```python
from build123d import *

# Parameters (mm, degrees)
F0_W     = 203.2
F0_H     = 127
F1_DEPTH = 127
F2_R     = 5.08
F3_W     = 152.4
F3_H     = 114.3
F4_DEPTH = 101.6
F3_W_2   = 31.75
F5_DEPTH = 6.35


with BuildPart() as f1:
    # F0 (on Top) → F1 (new body)
    with BuildSketch(Plane.XY):
        with Locations((38.395604, 24.034617)):
            Rectangle(F0_W, F0_H)
    extrude(amount=F1_DEPTH)

    # F2
    f2_edges = [f1.edges().sort_by_distance(p)[0] for p in [
        (38.395604, -39.465383, 127),
        (-63.204396, 24.034617, 127),
        (139.995604, 24.034617, 127),
        (139.995604, -39.465383, 63.5),
        (-63.204396, -39.465383, 63.5),
    ]]
    fillet(f2_edges, radius=F2_R)

    # F3 (on face) → F4 (cut)
    with BuildSketch(Plane.XZ.offset(39.465383)):
        with Locations((56.842002, 63.221574)):
            Rectangle(F3_W, F3_H)
    extrude(amount=-F4_DEPTH, mode=Mode.SUBTRACT)

    # F3 (on face) → F5 (cut)
    with BuildSketch(Plane.XZ.offset(39.465383)):
        with Locations((56.842002, 63.221574)):
            Rectangle(F3_W, F3_H)
        with Locations((-39.926485, 63.221574)):
            Rectangle(F3_W_2, F3_H)
    extrude(amount=-F5_DEPTH, mode=Mode.SUBTRACT)


solid = f1.part
```
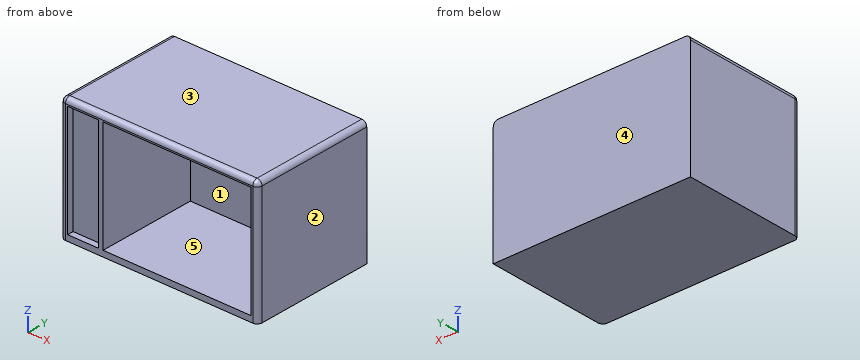
Check sheet for the modelled part. Datum: model origin and axes. Units: mm. Face numbers are marked on the shaded views. A direction names the side the tool comes from. Give positions to 0.01 mm unless a question says otherwise; leave off trailing zeros. Order: outer loops, then holes, each group sorted by start corner. A loop starts at its lowest first (then second) coordinate and runs counter-clockwise, first axis right, second up. Notation, with made-up numbers: (-2, 49.5) -> (47, 49.5) arc R31 cw to (47, 85.5) -> close; hole circle Ø8 at (79, 69.25). An arc over 180 degrees is marked (long way). Use CSV: the item, a comma, the result in double quotes. Start each with the question number.
1) Mould release check, pull along Z, two halves, no side actions. Record for the marked faces 1, 2 and 3: released by +Z, released by -Z, zero draft, split by the parting line, or undercut.
2) Sectioned sample at B-B, the plane x = -38. Record the boundary of the cut face in (y, z).
3) Go/stop test with flat-tipped pins: P1, Ø1.9, axis at x = -42, y = -36, coming from the +Z side; P2, Ø16, axis at x = -37, z = 89.5, coming from the -Y side; P3, Ø8, axis at x = 94, z = 42, coming from the -Y side. Record where each tip stops, or that it passes through.
4) Sectioned sample at C-C, the plane z = 22. Record the boundary of the cut face in (x, y).
5) Sectioned sample at D-D, the plane x = 36. Record the boundary of the cut face in (y, z).
6) Material ranges on line 1 (X direction, y = -12.5, z = 34); line 2 (Z direction, x = 11, y = 24); line 3 (Y direction, x = 39.5, z = 41), recorded low to high. Write a range as from..to.
7) Sectioned sample at A-A, the plane y = -22. Record the boundary of the cut face in (x, z), plus the area to 3 significant figures.
8) Set-up check for the marked faces 4 and 5: record each of +Z, -Z, +X, -X, +Y, -Y from which the full face is reachable in a straight line by a thin tool's end or side.
Recorded:
1,face 1,"undercut"
1,face 2,"zero draft"
1,face 3,"released by +Z"
2,outline,"(-39.47, 0) -> (87.53, 0) -> (87.53, 127) -> (-34.39, 127) arc R5.08 ccw to (-39.47, 121.92) -> (-39.47, 120.37) -> (-33.12, 120.37) -> (-33.12, 6.07) -> (-39.47, 6.07) -> close"
3,P1,"z = 126.96"
3,P2,"y = -33.12"
3,P3,"y = 62.13"
4,outline,"(-63.2, -34.39) arc R5.08 ccw to (-58.12, -39.47) -> (-55.8, -39.47) -> (-55.8, -33.12) -> (-24.05, -33.12) -> (-24.05, -39.47) -> (-19.36, -39.47) -> (-19.36, 62.13) -> (133.04, 62.13) -> (133.04, -39.47) -> (134.92, -39.47) arc R5.08 ccw to (140, -34.39) -> (140, 87.53) -> (-63.2, 87.53) -> close"
5,outline,"(-39.47, 0) -> (87.53, 0) -> (87.53, 127) -> (-34.39, 127) arc R5.08 ccw to (-39.47, 121.92) -> (-39.47, 120.37) -> (62.13, 120.37) -> (62.13, 6.07) -> (-39.47, 6.07) -> close"
6,line 1,"-63.2..-19.36, 133.04..140"
6,line 2,"0..6.07, 120.37..127"
6,line 3,"62.13..87.53"
7,outline,"(-63.2, 0) -> (140, 0) -> (140, 121.92) arc R5.08 ccw to (134.92, 127) -> (-58.12, 127) arc R5.08 ccw to (-63.2, 121.92) -> close; hole (-19.36, 6.07) -> (133.04, 6.07) -> (133.04, 120.37) -> (-19.36, 120.37) -> close"
7,area,"8,380 mm2"
8,face 4,"+Z, -Z, +X, -X, +Y"
8,face 5,"-Y"
